Job drawing, mm, ordinate dimensions from the low corner. One solid piece. A direction names the side the tool comes from. Coordinates: 2 decimals unless noted, no trailing zeros. Write each loop counter-clockwise with the first axis right and the second up, starting at its lowest first coordinate (ties: lowest second). Pieces come first, ordered by that corner, then holes. Notation, with made-up numbers: M 48,50.25 L 96,50.25 A18 ccw 96,61.25 Z; hole C 22,-25.75 d11. An arc over 180 degrees is marked long. Answer as CSV lines item,"result". Start each with the question number.
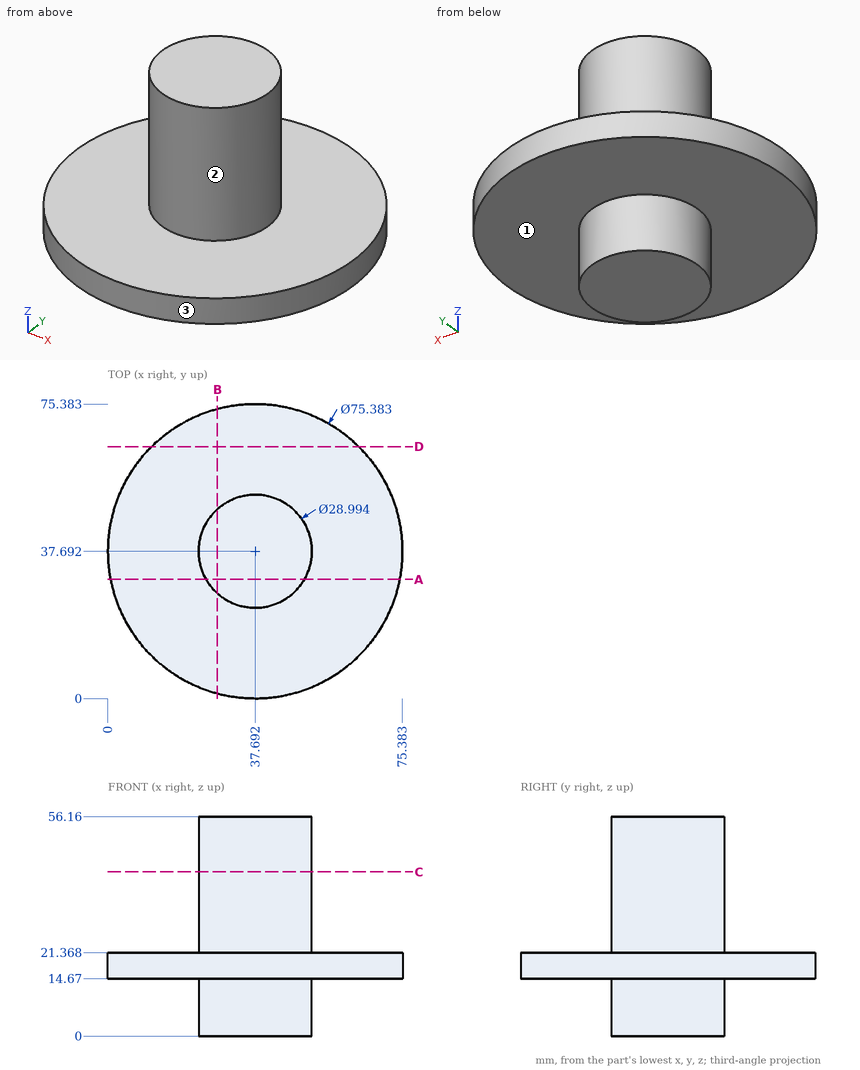
1) Band-saw the part on D-D, the plane y = 64.5. List the corners of the cut face in (x, z).
2) Probe L1, parallel to Z at x = 34, y = 9; L2, parallel to Y at x = 37, z = 48.5; L3, parallel to Y at x = 43, z = 34. List the from-to ranges inside material, lowest first. Write a range as [from, to].
3) Band-saw the part on C-C, the plane z = 42. List the corners of the cut face in (x, y), plus the area to 3 significant figures.
4) Tool access for the marked faces 1, 2 and 3: list every direction of +Z, -Z, +X, -X, +Y, -Y with a clear straight run to the whole face (end or side of a thin tool).
5) Band-saw the part on B-B, the plane x = 28. List the corners of the cut face in (y, z) (1 decimal), plus the area to 3 significant figures.
6) Band-saw the part on A-A, the plane y = 30.5. List the corners of the cut face in (x, z) (1 decimal).
7) Pin check, flat tips, straight feed: P1, Ø5, axis at y = 47.5, z = 27.5, coming from the -X side; P2, Ø6, axis at x = 16, y = 60, coming from the -Z side; P3, Ø1.5, axis at y = 51.5, z = 32.5, coming from the -X side (1 decimal). Stop position of each tip, or through.
Result sheet:
1,outline,"M 11.2,14.67 L 64.19,14.67 L 64.19,21.37 L 11.2,21.37 Z"
2,L1,"z = [14.67, 21.37]"
2,L2,"y = [23.21, 52.17]"
2,L3,"y = [24.2, 51.18]"
3,outline,"C 37.69,37.69 d28.99"
3,area,"660 mm²"
4,face 1,"-Z"
4,face 2,"+Z"
4,face 3,"+Z, -Z"
5,outline,"M 1.3,14.7 L 26.9,14.7 L 26.9,0 L 48.5,0 L 48.5,14.7 L 74.1,14.7 L 74.1,21.4 L 48.5,21.4 L 48.5,56.2 L 26.9,56.2 L 26.9,21.4 L 1.3,21.4 Z"
5,area,"1,550 mm²"
6,outline,"M 0.7,14.7 L 25.1,14.7 L 25.1,0 L 50.3,0 L 50.3,14.7 L 74.7,14.7 L 74.7,21.4 L 50.3,21.4 L 50.3,56.2 L 25.1,56.2 L 25.1,21.4 L 0.7,21.4 Z"
7,P1,"stops at x = 25.17"
7,P2,"stops at z = 14.67"
7,P3,"stops at x = 31.4"
